```python
from build123d import *

# Parameters (mm, degrees)
SKETCH1_R               = 4.85
BOSS_EXTRUDE1_DEPTH     = 345.867201
CUT_EXTRUDE1_DEPTH      = 346.935204522
CUT_EXTRUDE1_DEPTH_BACK = 346.935204522
SKETCH2_R               = 1.25
SCALE1_SCALE            = 1.5


with BuildPart() as part:
    # Sketch1 → Boss-Extrude1 (new body)
    with BuildSketch(Plane(origin=(0, 0, 0), x_dir=(0, 0, -1), z_dir=(1, 0, 0))):
        Circle(SKETCH1_R)
    extrude(amount=BOSS_EXTRUDE1_DEPTH)

    # Sketch2 → Cut-Extrude1 (cut, two sides: drawn at the far end of the back side and taken through both)
    with BuildSketch(Plane(origin=(0, 0, 0), x_dir=(1, 0, 0), z_dir=(0, 1, 0)).offset(-CUT_EXTRUDE1_DEPTH_BACK)):
        with Locations(Location((343.367201, 0, 0), (0, 0, 270))):
            Circle(SKETCH2_R)
    extrude(amount=CUT_EXTRUDE1_DEPTH + CUT_EXTRUDE1_DEPTH_BACK, mode=Mode.SUBTRACT)


with BuildPart() as part_1:
    # Scale1: scaled about (172.618275836, 0, 1.121e-06)
    add(part.part.scale(SCALE1_SCALE).moved(Location((-86.309137918, 0, -5.6e-07))))


solid = part_1.part
```
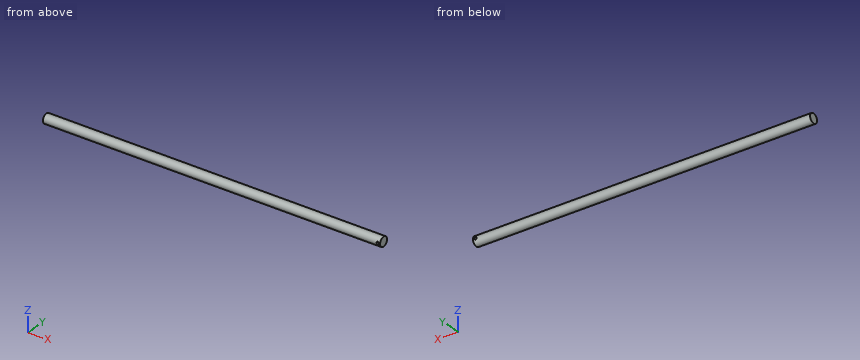
Check sheet for the modelled part. Datum: model origin and axes. Units: mm. Round coordinates to 2 decimals unless told otherwise and drop trailing zeros. Loops run counter-clockwise (first coordinate to the right, second up) from the corner with the lowest first, then second, coordinate; pieces in that order, holes last. Notation, with made-up numbers: (75.25, 80) - (96.25, 80) arc R20 cw to (96.25, 115) - close; hole circle Ø8 at (-6, 24). An arc over 180 degrees is marked (long way). Answer as a JSON object with one key per item and string values. Group by question number.
Q1. Gauge pin test, flat ends, axial feed: P1, Ø1, axis at x = 210, y = 3, coming from the -Z side; P2, Ø6, axis at x = 306, z = -5, coming from the -Y side; P3, Ø4, axis at x = 292, z = 5.5, coming from the -Y side. Record the tip position at first contact, or that the pin passes through.
Q2. Sectioned sample at A-A, the plane x = 334. Enter the section's corners in (y, z) (3 decimals), plus the area to 3 significant figures.
Q3. Scan lines: line 1 along X through (y, z) = (-2, 0); line 2 along X through (y, z) = (4, -0.5); line 3 along Z through (x, y) = (1, -5.5). Record each from-to range of solid material in increasing order. Write a range as [from, to].
Q4. Sectioned sample at C-C, the plane z = 5. Enter the section's corners in (x, y).
Q5. Sectioned sample at B-B, the plane y = -4. Enter the section's corners in (x, z) (3 decimals).
Solution:
{
 "1": {"P1": "stops at z = -6.83", "P2": "stops at y = -6.99", "P3": "stops at y = -6.38"},
 "2": {"outline": "circle Ø14.55 at (0, 0)", "area": "166 mm²"},
 "3": {"line 1": "x = [-86.31, 426.87], [430.62, 432.49]", "line 2": "x = [-86.31, 426.93], [430.55, 432.49]", "line 3": "z = [-4.76, 4.76]"},
 "4": {"outline": "(-86.31, -5.28) - (432.49, -5.28) - (432.49, 5.28) - (-86.31, 5.28) - close"},
 "5": {"outline": "(-86.309, -6.077) - (432.492, -6.077) - (432.492, 6.077) - (-86.309, 6.077) - close; hole circle Ø3.75 at (428.742, 0)"}
}
